The model under review builds one solid part; all positions refer to its coordinate system, in mm. A direction names the side the tool comes from. Round coordinates to 2 decimals unless told otherwise and drop trailing zeros. Write each loop counter-clockwise with the first axis right and the second up, starting at its lowest first coordinate (ties: lowest second). Pieces come first, ordered by that corner, then holes. Notation, with made-up numbers: (88.5, -31) - (134.5, -31) arc R17 cw to (134.5, -3) - close; hole circle Ø7 at (-5.5, -14.75). An arc over 180 degrees is marked (long way). Use one line per item in the form item = value.
from build123d import *

# Parameters (mm, degrees)
F1_DEPTH  = 71
F2_R      = 25
F4_DEPTH  = 849.526
F8_R      = 10
F9_DEPTH  = 853.624132
F10_R     = 10
F11_DEPTH = 853.624132


with BuildPart() as f1:
    # F0 (on Top) → F1 (new body)
    with BuildSketch(Plane.XY):
        with BuildLine():
            Line((844.948384, 88.06222), (835.474697, 87.074853))
            ThreePointArc((835.474697, 87.074853), (840, 0), (835.474697, -87.074853))
            Line((835.474697, -87.074853), (844.948384, -88.06222))
            ThreePointArc((844.948384, -88.06222), (849.525, 0), (844.948384, 88.06222))
        make_face()
    extrude(amount=F1_DEPTH)

    # F2
    f2_edges = [f1.edges().sort_by_distance(p)[0] for p in [
        (840.211541, -87.568536, 0),
        (840.211541, 87.568536, 0),
    ]]
    fillet(f2_edges, radius=F2_R)

    # F3 (on Right) → F4 (cut, through all)
    with BuildSketch(Plane.YZ):
        with BuildLine():
            Line((-53.95, 61.595), (53.95, 61.595))
            ThreePointArc((53.95, 61.595), (60.70287, 64.39213), (63.5, 71.145))
            Line((63.5, 71.145), (63.5, 188.595))
            Line((63.5, 188.595), (-63.5, 188.595))
            Line((-63.5, 188.595), (-63.5, 71.145))
            ThreePointArc((-63.5, 71.145), (-60.70287, 64.39213), (-53.95, 61.595))
        make_face()
    extrude(amount=F4_DEPTH, mode=Mode.SUBTRACT)

    # F8 (on face) → F9 (cut, through all)
    with BuildSketch(Plane(origin=(0, 0, 0), x_dir=(-0.070627, -0.997503, 0), z_dir=(-0.997503, 0.070627, 0))):
        with Locations((0, 23.569)):
            Circle(F8_R)
    extrude(amount=-F9_DEPTH, mode=Mode.SUBTRACT)

    # F10 (on face) → F11 (cut, through all)
    with BuildSketch(Plane(origin=(0, 0, 0), x_dir=(0.070627, -0.997503, 0), z_dir=(-0.997503, -0.070627, 0))):
        with Locations((0, 23.569)):
            Circle(F10_R)
    extrude(amount=-F11_DEPTH, mode=Mode.SUBTRACT)


solid = f1.part
(1) To check wall thickness, follow L1, parallel to X at y = -6, z = 38; L2, parallel to Z at x = 843, y = -44 (3 decimals); L3, parallel to Z at x = 839.25, y = 74. State the ranges of each line that lie inside material, in increasing order.
Geometry results:
L1 = 839.98 to 849.5
L2 = 0 to 61.595
L3 = 2.86 to 71
(2) Machinability: for faces 1 (the cylindrical face through (842.632, -60.725, 64.414)), 2 (the cylindrical face through (849.524, -1.235, 35.003)), which of the approach directions +Z, -Z, +X, -X, +Y, -Y give a long, thin tool a straight path to every point of the face, cutting with its end or side? Answer none if there is none.
Geometry results:
face_1 = +Z, +X, -X
face_2 = +Z, -Z, +X
(3) Add section A-A on z = 20.5. Write out the cut boundary in (x, y), then the cut area to 3 significant figures.
Geometry results:
outline = (835.52, -86.67) - (844.99, -87.66) arc R849.53 ccw to (846.68, -69.49) - (837.18, -68.82) arc R840 cw to start; (835.52, 86.67) arc R840 cw to (837.18, 68.82) - (846.68, 69.49) arc R849.53 ccw to (844.99, 87.66) - close; (838.52, -49.83) - (848.02, -50.5) arc R849.53 ccw to (848.02, 50.5) - (838.52, 49.83) arc R840 cw to start
area = 1,300 mm2
(4) Add section C-C on y = 35. Write out the cut boundary in (x, z) (3 decimals).
Geometry results:
outline = (839.271, 0) - (848.804, 0) - (848.804, 61.595) - (839.271, 61.595) - close
(5) Insertion check: P1, Ø3.5, axis at x = 845.5, y = 2, coming from the +Z side (3 decimals); P2, Ø1.5, axis at y = -56.5, z = 35.5, coming from the -X side; P3, Ø4, axis at y = -31.5, z = 28.5, coming from the -X side. Each pin has a flat end and moves straight along its axis. Give the tip position at first contact, or say it passes through.
Geometry results:
P1 = 61.595
P2 = 838.05
P3 = 839.33
(6) Add section B-B on z = 42.5. Write out the cut boundary in (x, y).
Geometry results:
outline = (835.47, -87.07) - (844.95, -88.06) arc R849.53 ccw to (844.95, 88.06) - (835.47, 87.07) arc R840 cw to start
(7) The part is to be moulded in two halves that separate along Y. For faces 3 (the flat face through (844, 1, 0)), 4 (the cylindrical face through (842.23, -64.26, 14.7)), 5 (the cylindrical face through (840.83, -80.47, 7.52)), say which applies: +Y half, -Y half, draft (parallel to the pull), parting line (faces both ways), or undercut.
Geometry results:
face_3 = draft
face_4 = undercut
face_5 = -Y half
(8) Add section D-D on x = 843. Count the separate pieces of the cut face and the enclosed holes in it, then the cut area to 3 significant figures.
Geometry results:
separate_pieces = 1
enclosed_holes = 2
area = 10,400 mm2
